The model under review builds one solid part; all positions refer to its coordinate system, in mm. A direction names the side the tool comes from. Coordinates: 2 decimals unless noted, no trailing zeros. Write each loop counter-clockwise with the first axis right and the second up, starting at its lowest first coordinate (ties: lowest second). Pieces come first, ordered by that corner, then holes. Notation, with made-up numbers: (31, 73.25) -> (57, 73.25) arc R17 ccw to (57, 89.25) -> close; hole circle Ø4 at (-15, -35). An arc over 180 degrees is marked (long way). Write each question's results on one line, items separated by ' | '.
```python
from build123d import *

# Parameters (mm, degrees)
EXTRUDE_1_DEPTH     = 3
SKETCH_2_R          = 1.6
CUT_EXTRUDE_1_DEPTH = 47.19523785
FILLET_1_R          = 5
SKETCH_3_R          = 2.1
CUT_EXTRUDE_2_DEPTH = 47.19523785


with BuildPart() as part:
    # 草图1 → 凸台-拉伸1 (new body)
    with BuildSketch(Plane(origin=(0, 0, 0), x_dir=(1, 0, 0), z_dir=(0, 1, 0))):
        Polygon((-30, 35), (-30, 15), (-10, 15), (-10, -15), (10, -15), (10, 35), align=None)
    extrude(amount=EXTRUDE_1_DEPTH)

    # 草图2 → 切除-拉伸1 (cut, through all)
    with BuildSketch(Plane(origin=(0, 3, 0), x_dir=(1, 0, 0), z_dir=(0, 1, 0))):
        with Locations(Location((-24.5, 29.5, 0), (0, 0, 270))):
            Circle(SKETCH_2_R)
        with Locations(Location((-24.5, 20.5, 0), (0, 0, 270))):
            Circle(SKETCH_2_R)
        with Locations(Location((-4.5, -9.5, 0), (0, 0, 270))):
            Circle(SKETCH_2_R)
        with Locations(Location((4.5, -9.5, 0), (0, 0, 270))):
            Circle(SKETCH_2_R)
    extrude(amount=-CUT_EXTRUDE_1_DEPTH, mode=Mode.SUBTRACT)

    # 圆角1
    fillet_1_edges = [part.edges().sort_by_distance(p)[0] for p in [
        (10, 1.5, 15),
        (-10, 1.5, 15),
        (-10, 1.5, -15),
        (-30, 1.5, -15),
        (-30, 1.5, -35),
        (10, 1.5, -35),
    ]]
    fillet(fillet_1_edges, radius=FILLET_1_R)

    # 草图3 → 切除-拉伸2 (cut, through all)
    with BuildSketch(Plane(origin=(0, 3, 0), x_dir=(1, 0, 0), z_dir=(0, 1, 0))):
        with Locations(Location((0, 25, 0), (0, 0, 270))):
            Circle(SKETCH_3_R)
    extrude(amount=-CUT_EXTRUDE_2_DEPTH, mode=Mode.SUBTRACT)


solid = part.part
```
Q1. Clearance check with a flat-ended pin moving along its axis: P1, Ø0.9, axis at x = -21, y = 1, coming from the +Z side. State where the tip first meets the part, or that it passes through.
Solution:
P1: z = -15
Q2. Machinability: for faces 1 (the flat face through (-20, 1, -15)), 2 (the flat face through (-30, 1, -25)), which of the approach directions +Z, -Z, +X, -X, +Y, -Y give a long, thin tool a straight path to every point of the face, cutting with its end or side? Answer none if there is none.
Solution:
face 1: +Z, -X, +Y, -Y | face 2: +Z, -Z, -X, +Y, -Y
Q3. For line 1 (X direction, y = 1, z = 9.5); line 2 (Z direction, x = -25.5, y = 1.7); line 3 (X direction, y = 1.25, z = -20.5), list the stretches that pass through material, from the lowest coordinate up. Write a range as from..to.
Solution:
line 1: -10..-6.1, -2.9..2.9, 6.1..10 | line 2: -34.97..-30.75, -28.25..-21.75, -19.25..-15.03 | line 3: -30..-26.1, -22.9..10
Q4. Add section C-C (y = 1.9). Write out the cut boundary in (x, z), plus the area to 3 significant figures.
Solution:
outline: (-30, -30) arc R5 ccw to (-25, -35) -> (5, -35) arc R5 ccw to (10, -30) -> (10, 10) arc R5 ccw to (5, 15) -> (-5, 15) arc R5 ccw to (-10, 10) -> (-10, -10) arc R5 cw to (-15, -15) -> (-25, -15) arc R5 ccw to (-30, -20) -> close; hole circle Ø3.2 at (-24.5, -29.5); hole circle Ø3.2 at (-24.5, -20.5); hole circle Ø3.2 at (-4.5, 9.5); hole circle Ø4.2 at (0, -25); hole circle Ø3.2 at (4.5, 9.5) | area: 1,330 mm²
Q5. Add section B-B (z = -25). Write out the cut boundary in (x, y), plus the area to 3 significant figures.
Solution:
outline: (-30, 0) -> (-2.1, 0) -> (-2.1, 3) -> (-30, 3) -> close; (2.1, 0) -> (10, 0) -> (10, 3) -> (2.1, 3) -> close | area: 107 mm²
Q6. Add section D-D (x = -9). Write out the cut boundary in (y, z), plus the area to 3 significant figures.
Solution:
outline: (0, -35) -> (3, -35) -> (3, 13) -> (0, 13) -> close | area: 144 mm²
Q7. Add section A-A (x = 0). Write out the cut boundary in (y, z), plus the area to 3 significant figures.
Solution:
outline: (0, -35) -> (3, -35) -> (3, -27.1) -> (0, -27.1) -> close; (0, -22.9) -> (3, -22.9) -> (3, 15) -> (0, 15) -> close | area: 137 mm²
Q8. Draft analysis for pull direction Z (two halves, no side actions). For faces 3 (the flat face through (-6, 3, -16)), 4 (the cylindrical face through (-9, 2, 13)), 5 (the cylindrical face through (-22.914, 1.521, -20.708)), state which applies: pulls with the +Z half, pulls with the -Z half, needs draft (parallel to the pull), parting line crosses it, or undercut.
Solution:
face 3: needs draft | face 4: pulls with the +Z half | face 5: undercut
